The model under review builds one solid part; all positions refer to its coordinate system, in mm. Face numbers are marked on the shaded views. A direction names the side the tool comes from. Give positions to 0.01 mm unless a question says otherwise; leave off trailing zeros. Loops run counter-clockwise (first coordinate to the right, second up) from the corner with the lowest first, then second, coordinate; pieces in that order, holes last. Notation, with made-up numbers: M -19.75,-7.5 L 16.25,-7.5 A20 ccw 16.25,10.5 Z; hole C -25.5,66 d2. An arc over 180 degrees is marked long. Write item = value, one per line. Start each with the question number.
1. Draft analysis for pull direction Z (two halves, no side actions). For the marked faces 3, 4 and 5, state which applies: pulls with the +Z half, pulls with the -Z half, needs draft (parallel to the pull), parting line crosses it, or undercut.
2. We need section C-C on x = -15.5. Give the boundary of the cut face in (y, z).
3. We need section D-D on z = 4. Count the separate pieces of the cut face and the enclosed holes in it, then the cut area to 3 significant figures.
4. Wall thickness on line 1 along X through (y, z) = (15.5, -3); line 2 along X through (y, z) = (8, 0); line 3 along Y through (x, z) = (-2.75, 0.25): over which ranges is each line inside the solid? List them lowest first. Write a range as from..to.
5. For pin 1 (5 mm diameter, centred on x = -13.5, z = -2, fed in from -Y); pin 2 (4 mm diameter, centred on x = -5.5, z = 4, fed in from -Y); pin 3 (3.5 mm diameter, centred on y = 12, z = 0, fed in from +X); pin 4 (1 mm diameter, centred on x = -12, y = 11.5, fed in from -Z), all flat-tipped, find the tip position at first contact; note any pin that passes through.
6. We need section B-B on y = 12. Give the boundary of the cut face in (x, z), then the cut area to 3 significant figures.
7. For the marked faces 1 and 2, list the 3-axis set-ups (+Z, -Z, +X, -X, +Y, -Y) from which the entire face can be reached by the end or side of a thin tool; tool diameter is ignored.
8. We need section A-A on z = 0. Give the boundary of the cut face in (x, y).
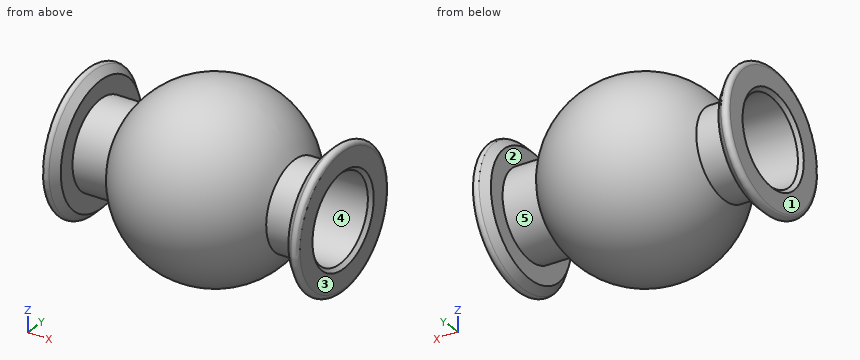
from build123d import *

# Parameters (mm, degrees)
SKETCH3_R          = 3
CUT_EXTRUDE4_DEPTH = 24


with BuildPart() as part:
    # Sketch2 → Revolve2 (revolve)
    with BuildSketch(Plane.XY, mode=Mode.PRIVATE) as revolve2_sk:
        with BuildLine():
            Line((-13.618675666, 15.043449319), (-16, 15.043449319))
            Line((-16, 15.043449319), (-16, 16.285660618))
            Line((-16, 16.285660618), (-16.497212995, 16.782873614))
            ThreePointArc((-16.497212995, 16.782873614), (-16.824150059, 16.847905439), (-17.00934503, 16.570741579))
            Line((-17.00934503, 16.570741579), (-17.00934503, 15.25))
            Line((-17.00934503, 15.25), (-16.504672515, 14.745327485))
            Line((-16.504672515, 14.745327485), (-16.504672515, 12))
            Line((-16.504672515, 12), (0.504672515, 12))
            Line((0.504672515, 12), (0.504672515, 14.745327485))
            Line((0.504672515, 14.745327485), (1.00934503, 15.25))
            Line((1.00934503, 15.25), (1.00934503, 16.570741579))
            ThreePointArc((1.00934503, 16.570741579), (0.824150059, 16.847905439), (0.497212995, 16.782873614))
            Line((0.497212995, 16.782873614), (0, 16.285660618))
            Line((0, 16.285660618), (0, 15.043449319))
            Line((0, 15.043449319), (-2.381324334, 15.043449319))
            ThreePointArc((-2.381324334, 15.043449319), (-8, 18.39), (-13.618675666, 15.043449319))
        make_face()
    revolve(revolve2_sk.sketch.rotate(Axis((-16.504672515, 12, 0), (1, 0, 0)), 90), axis=Axis((-16.504672515, 12, 0), (1, 0, 0)))

    # Sketch3 → Cut-Extrude4 (cut)
    with BuildSketch(Plane(origin=(1.00934503, 0, 0), x_dir=(0, 0, -1), z_dir=(1, 0, 0))):
        with Locations((0, 12)):
            Circle(SKETCH3_R)
    extrude(amount=-CUT_EXTRUDE4_DEPTH, mode=Mode.SUBTRACT)


solid = part.part
Final values:
q1.face_3 = needs draft
q1.face_4 = undercut
q1.face_5 = parting line crosses it
q2.outline = C 12,0 d6.09; hole C 12,0 d6
q3.separate_pieces = 3
q3.enclosed_holes = 0
q3.area = 87.7 mm²
q4.line_1 = -17.01..-16.32, -12.43..-3.57, 0.32..1.01
q4.line_2 = -17.01..-16, -12.98..-3.02, 0..1.01
q4.line_3 = 8.37..9.01, 14.99..15.63
q5.pin_1 = 6.56
q5.pin_2 = 6.22
q5.pin_3 = through
q5.pin_4 = -5.33
q6.outline = M -17.01,-4.57 A0.3 ccw -16.5,-4.78 L -16,-4.29 L -16,-3.04 L -13.62,-3.04 A6.39 ccw -2.38,-3.04 L 0,-3.04 L 0,-4.29 L 0.5,-4.78 A0.3 ccw 1.01,-4.57 L 1.01,-3.25 L 0.76,-3 L -16.76,-3 L -17.01,-3.25 Z; M -17.01,3.25 L -16.76,3 L 0.76,3 L 1.01,3.25 L 1.01,4.57 A0.3 ccw 0.5,4.78 L 0,4.29 L 0,3.04 L -2.38,3.04 A6.39 ccw -13.62,3.04 L -16,3.04 L -16,4.29 L -16.5,4.78 A0.3 ccw -17.01,4.57 Z
q6.area = 61.6 mm²
q7.face_1 = +Z, -Z, -X, +Y, -Y
q7.face_2 = none
q8.outline = M -17.01,7.43 A0.3 ccw -16.5,7.22 L -16,7.71 L -16,8.96 L -13.62,8.96 A6.39 ccw -2.38,8.96 L 0,8.96 L 0,7.71 L 0.5,7.22 A0.3 ccw 1.01,7.43 L 1.01,8.75 L 0.76,9 L -16.76,9 L -17.01,8.75 Z; M -17.01,15.25 L -16.76,15 L 0.76,15 L 1.01,15.25 L 1.01,16.57 A0.3 ccw 0.5,16.78 L 0,16.29 L 0,15.04 L -2.38,15.04 A6.39 ccw -13.62,15.04 L -16,15.04 L -16,16.29 L -16.5,16.78 A0.3 ccw -17.01,16.57 Z
